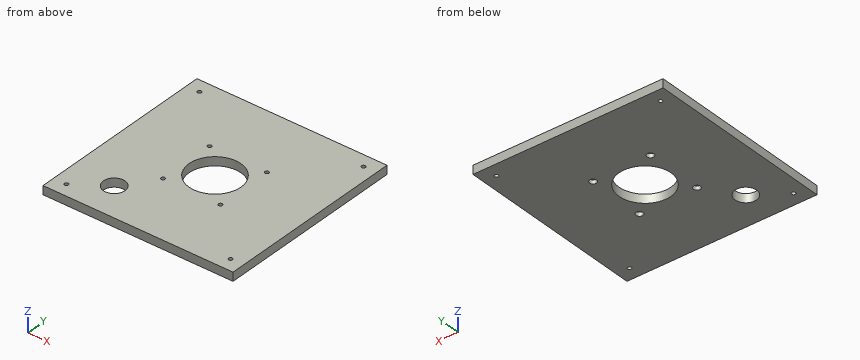
```python
from build123d import *

# Parameters (mm, degrees)
SK_PLACA_W                         = 220
SK_PLACA_H                         = 220
PLACA_DEPTH                        = 10
SK_PASO_CABLES_R                   = 30
PASO_CABLES_DEPTH                  = 10
SK_PASANTES_M4_PEDESTAL_R          = 2.25
PASANTES_M4_PEDESTAL_DEPTH         = 10
SK_CAJAS_M4_INFERIORES_R           = 4
CAJAS_M4_INFERIORES_DEPTH          = 4.5
SK_PASANTES_M4_SEPARADORES_CAJA_R  = 2.25
PASANTES_M4_SEPARADORES_CAJA_DEPTH = 10
SK_PASO_CABLES_CAJA_R              = 12.5
PASO_CABLES_CAJA_DEPTH             = 10


with BuildPart() as part:
    # Sk_Placa → Placa (new body)
    with BuildSketch(Plane.XY):
        Rectangle(SK_PLACA_W, SK_PLACA_H)
    extrude(amount=PLACA_DEPTH)

    # Sk_Paso_cables → Paso_cables (cut)
    with BuildSketch(Plane.XY):
        Circle(SK_PASO_CABLES_R)
    extrude(amount=PASO_CABLES_DEPTH, mode=Mode.SUBTRACT)

    # Sk_Pasantes_M4_pedestal → Pasantes_M4_pedestal (cut)
    with BuildSketch(Plane.XY):
        with Locations((33.234018716, 33.234018716)):
            Circle(SK_PASANTES_M4_PEDESTAL_R)
        with Locations((-33.234018716, 33.234018716)):
            Circle(SK_PASANTES_M4_PEDESTAL_R)
        with Locations((-33.234018716, -33.234018716)):
            Circle(SK_PASANTES_M4_PEDESTAL_R)
        with Locations((33.234018716, -33.234018716)):
            Circle(SK_PASANTES_M4_PEDESTAL_R)
    extrude(amount=PASANTES_M4_PEDESTAL_DEPTH, mode=Mode.SUBTRACT)

    # Sk_Cajas_M4_inferiores → Cajas_M4_inferiores (cut)
    with BuildSketch(Plane.XY):
        with Locations((33.234018716, 33.234018716)):
            Circle(SK_CAJAS_M4_INFERIORES_R)
        with Locations((-33.234018716, 33.234018716)):
            Circle(SK_CAJAS_M4_INFERIORES_R)
        with Locations((-33.234018716, -33.234018716)):
            Circle(SK_CAJAS_M4_INFERIORES_R)
        with Locations((33.234018716, -33.234018716)):
            Circle(SK_CAJAS_M4_INFERIORES_R)
    extrude(amount=CAJAS_M4_INFERIORES_DEPTH, mode=Mode.SUBTRACT)

    # Sk_Pasantes_M4_separadores_caja → Pasantes_M4_separadores_caja (cut)
    with BuildSketch(Plane.XY):
        with Locations((-95, -95)):
            Circle(SK_PASANTES_M4_SEPARADORES_CAJA_R)
        with Locations((-95, 95)):
            Circle(SK_PASANTES_M4_SEPARADORES_CAJA_R)
        with Locations((95, -95)):
            Circle(SK_PASANTES_M4_SEPARADORES_CAJA_R)
        with Locations((95, 95)):
            Circle(SK_PASANTES_M4_SEPARADORES_CAJA_R)
    extrude(amount=PASANTES_M4_SEPARADORES_CAJA_DEPTH, mode=Mode.SUBTRACT)

    # Sk_Paso_cables_caja → Paso_cables_caja (cut)
    with BuildSketch(Plane.XY):
        with Locations((-60, -70)):
            Circle(SK_PASO_CABLES_CAJA_R)
    extrude(amount=PASO_CABLES_CAJA_DEPTH, mode=Mode.SUBTRACT)


solid = part.part
```
Can you work these out from the model? Positions are in its coordinate system, mm. Give positions to 0.01 mm unless a question says otherwise; leave off trailing zeros. Loops run counter-clockwise (first coordinate to the right, second up) from the corner with the lowest first, then second, coordinate; pieces in that order, holes last. Notation, with made-up numbers: M 12,15 L 64,15 A17 ccw 64,47 Z; hole C -24.75,12 d7. An arc over 180 degrees is marked long. Use one line per item in the form item = value. Start each with the question number.
(1) I'm going to push flat-ended pins straight in: P1, Ø6.5, axis at x = 33.23, y = 33.23, coming from the -Z side; P2, Ø4, axis at x = -95, y = 95, coming from the -Z side. Where does each tip first touch, or does it pass through?
(2) Please list where these lines run through material, in increasing order: line 1 (Y direction, x = -95, z = 3.5); line 2 (X direction, y = -33, z = 6.5); line 3 (X direction, y = -18, z = 6).
(3) I want a section at C-C, the plane z = 6.5. State how many separate pieces and enclosed holes the cut face has, and give its area (3 significant figures).
(4) I want a section at A-A, the plane x = 0. Write out the boundary of the cut face in (y, z).
(5) I want a section at B-B, the plane y = -70. Write out the boundary of the cut face in (x, z), and give its area (3 significant figures).
Worked out:
q1.P1 = 4.5
q1.P2 = through
q2.line_1 = -110 to -97.25, -92.75 to 92.75, 97.25 to 110
q2.line_2 = -110 to -35.47, -31 to 31, 35.47 to 110
q2.line_3 = -110 to -24, 24 to 110
q3.separate_pieces = 1
q3.enclosed_holes = 10
q3.area = 45,000 mm²
q4.outline = M -110,0 L -30,0 L -30,10 L -110,10 Z; M 30,0 L 110,0 L 110,10 L 30,10 Z
q5.outline = M -110,0 L -72.5,0 L -72.5,10 L -110,10 Z; M -47.5,0 L 110,0 L 110,10 L -47.5,10 Z
q5.area = 1,950 mm²
